Source: three-view drawing plus pictorial views. Frame: mm from the lowest corner of the part. Give positions to 0.01 mm unless a question says otherwise; leave off trailing zeros. Write each loop counter-clockwise with the first axis right and the second up, starting at its lowest first coordinate (ties: lowest second). Pieces come first, ordered by that corner, then holes.
Q1. Draft query along Y for the marked faces 1 and 2. Return one class per face: pulls with the +Y half, pulls with the -Y half, needs draft (parallel to the pull), parting line crosses it, or undercut.
Q2. Cut plane D-D on y = 5.25. Return the cut outline in (x, z).
Q3. Line query: L1, parallel to X at y = 2.5, z = 7.5; L2, parallel to Y at x = 39, z = 6; L3, parallel to Y at x = 47.5, z = 3.75. Output: solid intervals per line, ascending.
Q4. Cut plane C-C on x = 68.5. Return the cut outline in (y, z), plus the area to 3 significant figures.
Q5. Pin query (flat end, axial travel): pin 1 (0.6 mm diameter, centred on y = 7.5, z = 3.5, fed in from +X); pin 2 (3 mm diameter, centred on x = 20.5, y = 5, fed in from +Z); pin 3 (1.5 mm diameter, centred on x = 60.5, z = 5.5, fed in from +Y); pin 4 (1 mm diameter, centred on x = 58.5, z = 3, fed in from +Y). Return the tip coordinate at first contact, or that it passes through.
Q6. Cut plane A-A on z = 3. Return the cut outline in (x, y), plus the area to 3 significant figures.
Q7. Cut plane B-B on y = 1.5. Return the cut outline in (x, z), plus the area to 3 significant figures.
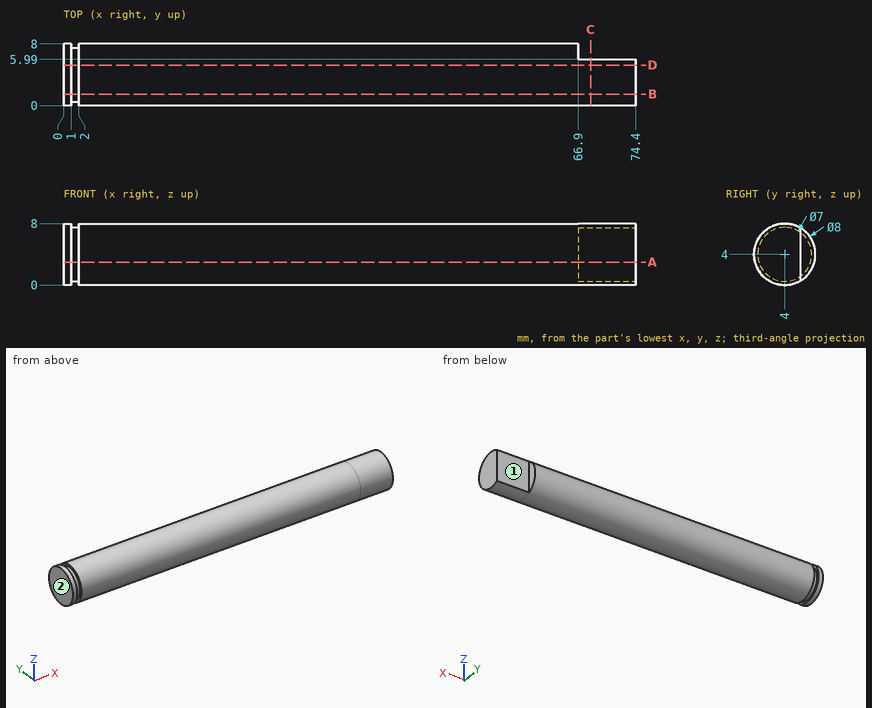
Data:
1. face 1: pulls with the +Y half
1. face 2: needs draft
2. outline: (0, 0.2) - (1, 0.2) - (1, 0.73) - (2, 0.73) - (2, 0.2) - (74.4, 0.2) - (74.4, 7.8) - (2, 7.8) - (2, 7.27) - (1, 7.27) - (1, 7.8) - (0, 7.8) - close
3. L1: x = 0 to 1, 2 to 74.4
3. L2: y = 0.54 to 7.46
3. L3: y = 0.01 to 7.99
4. outline: (5.99, 0.53) - (5.99, 7.47) arc R4 ccw (long way) to start
4. area: 40.4 mm2
5. pin 1: stops at x = 66.9
5. pin 2: stops at z = 8
5. pin 3: stops at y = 7.93
5. pin 4: stops at y = 7.97
6. outline: (0, 0.13) - (1, 0.13) - (1, 0.65) - (2, 0.65) - (2, 0.13) - (74.4, 0.13) - (74.4, 5.99) - (66.9, 5.99) - (66.9, 7.87) - (2, 7.87) - (2, 7.35) - (1, 7.35) - (1, 7.87) - (0, 7.87) - close
6. area: 561 mm2
7. outline: (0, 0.88) - (1, 0.88) - (1, 1.55) - (2, 1.55) - (2, 0.88) - (74.4, 0.88) - (74.4, 7.12) - (2, 7.12) - (2, 6.45) - (1, 6.45) - (1, 7.12) - (0, 7.12) - close
7. area: 463 mm2
